Check sheet for the modelled part. Datum: model origin and axes. Units: mm. Give positions to 0.01 mm unless a question says otherwise; leave off trailing zeros. Write each loop counter-clockwise with the first axis right and the second up, starting at its lowest first coordinate (ties: lowest second). Pieces come first, ordered by that corner, then holes. Notation, with made-up numbers: (60, 24.5) -> (111, 24.5) arc R13 ccw to (111, 43.5) -> close; hole circle Ø11 at (-14.5, -19). An arc over 180 degrees is marked (long way). Return JSON: item names as keys, results as strings.
Autodesk Inventor part; units mm, degrees
ref_plane "YZ Plane" through (0, 0, 0) normal (1, 0, 0) x (0, 1, 0)
ref_plane "XZ Plane" through (0, 0, 0) normal (0, 1, 0) x (-1, 0, 0)
ref_plane "XY Plane" through (0, 0, 0) normal (0, 0, 1) x (1, 0, 0)
sketch "スケッチ1" plane through (0, 0, 0) normal (0, 0, 1) x (1, 0, 0)
  circle A0 centre (2.8, 0) radius 2.8
  line L0 (2.8, 0) -> (0, 0)
  circle A1 centre (0, 2.8) radius 2.8
  circle A2 centre (-2.8, 0) radius 2.8
  circle A3 centre (0, -2.8) radius 2.8
  circle A4 centre (2.8, 0) radius 1.5
  circle A5 centre (0, 2.8) radius 1.5
  circle A6 centre (-2.8, 0) radius 1.5
  circle A7 centre (0, -2.8) radius 1.5
  circle A8 centre (0, 0) radius 5
  circle A9 centre (0, 5) radius 1.5
  circle A10 centre (-5, 0) radius 1.5
  circle A11 centre (0, -5) radius 1.5
  circle A12 centre (5, 0) radius 1.5
  point P0 (-1.483, -4.775)
  point P1 (1.483, -4.775)
  point P2 (-4.775, -1.483)
  point P3 (-4.775, 1.483)
  point P4 (4.775, 1.483)
  point P5 (4.775, -1.483)
  point P6 (-1.483, 4.775)
  point P7 (1.483, 4.775)
  dimension "d12" = 10
  dimension "d1" = 5.6
  dimension "d4" = 360
  dimension "d7" = 3
  dimension "d10" = 360
  dimension "d15" = 3
  dimension "d18" = 360
extrude "押し出し1" add sketch "スケッチ1" along normal blind 3 contours A8 A12 A4 A1 A0 | A0 A1 A8 | A8 A12 A4 | A8 A3 A0 | A0 A3 A4 A12 A8 | A1 A4 A0 A5 | A0 A5 A9 A8 A1 | A3 A8 A11 A7 A0 | A0 A7 A3 A4 | A9 A5 A8 | A8 A11 A7 | A0 A2 A5 | A4 L0 A1 | A9 A5 A2 A1 A8 | A7 A2 A0 | A3 L0 A4 | A8 A3 A2 A7 A11 | A3 A6 A1 | A1 A6 A2 A5 | A2 A7 A3 A6 | A1 A2 A8 | A8 A2 A3 | A1 A6 A10 A8 A2 | A2 A8 A10 A6 A3 | A10 A6 A8
properties part number "カムL3" material "アセタール樹脂、白"
(1) Cross-section at B-B on x = -2.25. Enter the section's corners in (y, z), then the cut area to 3 significant figures.
Reply:
{"outline": "(-4.47, 0) -> (-1.4, 0) -> (-1.4, 3) -> (-4.47, 3) -> close; (1.4, 0) -> (4.47, 0) -> (4.47, 3) -> (1.4, 3) -> close", "area": "18.4 mm^2"}
(2) Thickness scan on L1, parallel to Y at x = 0, z = 1.3; L2, parallel to X at y = -0.5, z = 1.05. Record the ranges inside material, lowest first.
Reply:
{"L1": "-5 to -4.3, -1.3 to 1.3, 4.3 to 5", "L2": "-4.97 to -4.21, -1.39 to 1.39, 4.21 to 4.97"}
(3) Cross-section at D-D on z = 0.85. Enter the section's corners in (x, y).
Reply:
{"outline": "circle Ø10 at (0, 0); hole circle Ø3 at (-2.8, 0); hole circle Ø3 at (0, -2.8); hole circle Ø3 at (0, 2.8); hole circle Ø3 at (2.8, 0)"}
(4) Release check for a two-part mould opening along Y. For faces 1 (the cylindrical face through (-0.325, -1.336, 1.479)), 2 (the cylindrical face through (-0.195, 1.313, 1.479)), 3 (the cylindrical face through (-1.08, 4.88, 1.48)), 4 (the flat face through (0, 0, 3)) record: pulls with the +Y half, pulls with the -Y half, needs draft (parallel to the pull), parting line crosses it, or undercut.
Reply:
{"face 1": "undercut", "face 2": "undercut", "face 3": "parting line crosses it", "face 4": "needs draft"}
(5) Cross-section at C-C on y = -4. Enter the section's corners in (x, z).
Reply:
{"outline": "(-3, 0) -> (-0.9, 0) -> (-0.9, 3) -> (-3, 3) -> close; (0.9, 0) -> (3, 0) -> (3, 3) -> (0.9, 3) -> close"}
(6) Cross-section at A-A on y = 0. Enter the section's corners in (x, z), then the cut area to 3 significant figures.
Reply:
{"outline": "(-5, 0) -> (-4.3, 0) -> (-4.3, 3) -> (-5, 3) -> close; (-1.3, 0) -> (1.3, 0) -> (1.3, 3) -> (-1.3, 3) -> close; (4.3, 0) -> (5, 0) -> (5, 3) -> (4.3, 3) -> close", "area": "12.0 mm^2"}
(7) Depth check by flat-ended pin: pin 1 Ø1.5 at (y, z) = (-2.5, 2) entering from +X. Enter the tip coordinate at first touch or a pass-through.
Reply:
{"pin 1": "x = 4.68"}
